```python
from build123d import *

# Parameters (mm, degrees)
SKETCH1_R           = 2
BOSS_EXTRUDE1_DEPTH = 10
BOSS_EXTRUDE1_TAPER = 4
SKETCH1_2_R         = 2
BOSS_EXTRUDE2_DEPTH = 17.5
FILLET1_R           = 1


with BuildPart() as part:
    # Sketch1 → Boss-Extrude1 (new body)
    with BuildSketch(Plane.XY):
        Circle(SKETCH1_R)
    extrude(amount=BOSS_EXTRUDE1_DEPTH, taper=BOSS_EXTRUDE1_TAPER)

    # Sketch1<2> → Boss-Extrude2 (add)
    with BuildSketch(Plane.XY):
        Circle(SKETCH1_2_R)
    extrude(amount=-BOSS_EXTRUDE2_DEPTH)

    # Fillet1
    fillet1_edges = [part.edges().sort_by_distance(p)[0] for p in [
        (-1.300731881, 0, 10),
    ]]
    fillet(fillet1_edges, radius=FILLET1_R)


solid = part.part
```
The listing builds one solid part. Answer for the finished solid, in the listing's coordinates (mm). Round coordinates to 2 decimals unless told otherwise and drop trailing zeros. Order: outer loops, then holes, each group sorted by start corner. A loop starts at its lowest first (then second) coordinate and runs counter-clockwise, first axis right, second up. Notation, with made-up numbers: (17, 44) -> (22, 44) arc R19 cw to (22, 64) -> close; hole circle Ø8 at (-17.75, 71). An arc over 180 degrees is marked (long way). Answer as CSV lines item,"result".
Q1. A cutting plane is placed at A-A on z = -15.5. Determine the outline of the cut face in (x, y), plus the area to 3 significant figures.
Computed values:
outline,"circle Ø4 at (0, 0)"
area,"12.6 mm^2"
Q2. Consider line 1 (X direction, y = 1.15, z = 3); line 2 (Y direction, x = -0.95, z = -2); line 3 (X direction, y = 1.5, z = -15). Determine where each line is inside the solid, lowest interval first. Write a range as from..to.
Computed values:
line 1,"x = -1.37..1.37"
line 2,"y = -1.76..1.76"
line 3,"x = -1.32..1.32"
Q3. A cutting plane is placed at B-B on z = 5.75. Determine the outline of the cut face in (x, y), plus the area to 3 significant figures.
Computed values:
outline,"circle Ø3.2 at (0, 0)"
area,"8.02 mm^2"
Q4. Given pin 1 (1 mm diameter, centred on x = -1.5, z = -12, fed in from +Y); pin 2 (1 mm diameter, centred on x = -1, z = -5.5, fed in from +Y); pin 3 (2 mm diameter, centred on x = 0, z = 4, fed in from -Y), each flat-ended and moving along its own axis, determine where each tip first touches the part or whether it passes through.
Computed values:
pin 1,"stops at y = 1.73"
pin 2,"stops at y = 1.94"
pin 3,"stops at y = -1.79"
